Source: three-view drawing plus pictorial views. Frame: mm from the lowest corner of the part. A direction names the side the tool comes from. Coordinates: 2 decimals unless noted, no trailing zeros. Loops run counter-clockwise (first coordinate to the right, second up) from the corner with the lowest first, then second, coordinate; pieces in that order, holes last. Notation, with made-up numbers: (10.25, 53.5) - (63.25, 53.5) arc R21 cw to (63.25, 69.5) - close; hole circle Ø4 at (32.5, -5.5). An arc over 180 degrees is marked (long way). Return JSON: item names as keys, results as strings.
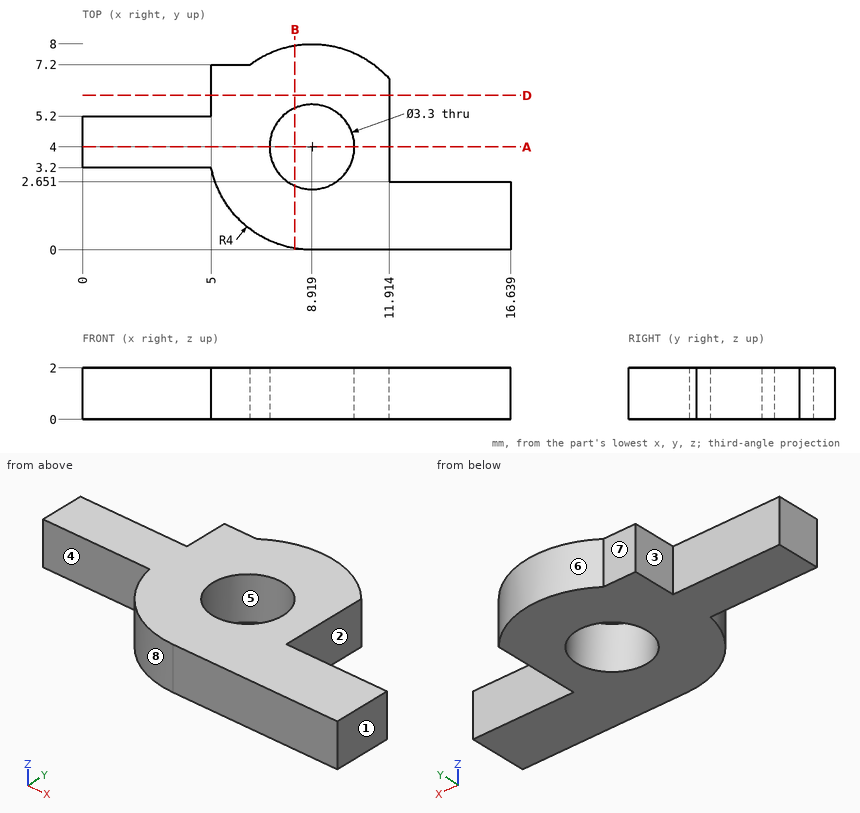
Item 1: Ray query, probe 1 along Y at (x, z) = (13.75, 1.9); probe 2 along X at (y, z) = (4.5, 1.85) (1 decimal); probe 3 along X at (y, z) = (3, 1.6) (1 decimal). Return the intervals inside material, ascending. Write a range as from..to.
Worked out:
{"probe 1": "0..2.65", "probe 2": "0..7.3, 10.5..11.9", "probe 3": "5..7.6, 10.2..11.9"}
Item 2: Section query B-B, the plane x = 8.25. Return loops of the section in (y, z).
Worked out:
{"outline": "(0.06, 0) - (2.49, 0) - (2.49, 2) - (0.06, 2) - close; (5.51, 0) - (7.94, 0) - (7.94, 2) - (5.51, 2) - close"}
Item 3: Reachability of the marked faces 1, 2, 3 and 4 from +Z, -Z, +X, -X, +Y, -Y: full face, straight path, thin tool, end or side. Return the list, or none.
Worked out:
{"face 1": "+Z, -Z, +X, +Y, -Y", "face 2": "+Z, -Z, +X, +Y", "face 3": "+Z, -Z, -X, +Y", "face 4": "+Z, -Z, -X, -Y"}
Item 4: Mould query, pull axis X, two halves, no side actions, for the marked faces 5, 6, 7 and 8. Classes: +X half, -X half, draft (parallel to the pull), parting line (faces both ways), or undercut.
Worked out:
{"face 5": "undercut", "face 6": "parting line", "face 7": "draft", "face 8": "-X half"}
Item 5: First-contact query: pin 1 Ø0.8 at (x, z) = (6, 0.5) entering from +Y. Flat tip, straight axial feed; report the tip coordinate or a pass-through.
Worked out:
{"pin 1": "y = 7.2"}
Item 6: Section query A-A, the plane y = 4. Return loops of the section in (x, z) (1 decimal).
Worked out:
{"outline": "(0, 0) - (7.3, 0) - (7.3, 2) - (0, 2) - close; (10.6, 0) - (11.9, 0) - (11.9, 2) - (10.6, 2) - close"}
Item 7: Section query D-D, the plane y = 6. Return loops of the section in (x, z) (1 decimal), and give its area (3 significant figures).
Worked out:
{"outline": "(5, 0) - (11.9, 0) - (11.9, 2) - (5, 2) - close", "area": "13.8 mm^2"}
